```python
from build123d import *

# Parameters (mm, degrees)
F0_R          = 12.7
F1_DEPTH      = 1.27
F1_DEPTH_BACK = 1.27
F0_W          = 2.54
F0_H          = 2.54
F2_DEPTH      = 10.16
F2_DEPTH_BACK = 10.16
F3_DEPTH      = 1.27
F3_DEPTH_BACK = 1.27
F4_DEPTH      = 1.27
F4_DEPTH_BACK = 1.27
F5_DEPTH      = 1.27
F5_DEPTH_BACK = 1.27
F6_DEPTH      = 1.27
F6_DEPTH_BACK = 1.27


# Not quite as in the source:
# - a feature of the source that left no trace in its solid (it failed there, or was rolled back) is left out
# - a pattern or mirror of a feature is missing from the dataset's text; its kind, count and spacing are read off the source's solid


with BuildPart() as f1:
    # F0 (on Right) → F1 (new body, two sides)
    with BuildSketch(Plane.YZ) as f1_sk:
        Circle(F0_R)
        with BuildLine():
            ThreePointArc((-10.0803124952, 1.27), (-7.1842048969, 7.1842048969), (-1.27, 10.0803124952))
            ThreePointArc((-1.27, 10.0803124952), (0, 10.16), (1.27, 10.0803124952))
            ThreePointArc((1.27, 10.0803124952), (7.1842048969, 7.1842048969), (10.0803124952, 1.27))
            ThreePointArc((10.0803124952, 1.27), (10.1400585538, 0.6362487914), (10.16, 0))
            ThreePointArc((10.16, 0), (10.1400585538, -0.6362487914), (10.0803124952, -1.27))
            ThreePointArc((10.0803124952, -1.27), (7.1842048969, -7.1842048969), (1.27, -10.0803124952))
            ThreePointArc((1.27, -10.0803124952), (0, -10.16), (-1.27, -10.0803124952))
            ThreePointArc((-1.27, -10.0803124952), (-7.1842048969, -7.1842048969), (-10.0803124952, -1.27))
            ThreePointArc((-10.0803124952, -1.27), (-10.16, 0), (-10.0803124952, 1.27))
        make_face(mode=Mode.SUBTRACT)
    extrude(amount=F1_DEPTH)
    extrude(f1_sk.sketch, amount=-F1_DEPTH_BACK)

    # F1_copies: F1 across plane


with BuildPart() as f1_1:
    add(f1.part)
    add(f1.part.mirror(Plane(origin=(0, 0, 0), x_dir=(0.7071067812, 0, -0.7071067812), z_dir=(0.7071067812, 0, 0.7071067812))))

    # F1_copies1: F1 across plane


with BuildPart() as f1_2:
    add(f1_1.part)
    add(f1_1.part.mirror(Plane(origin=(0, 0, 0), x_dir=(-0.7071067812, 0.7071067812, 0), z_dir=(-0.7071067812, -0.7071067812, 0))))

    # F0 (on Right) → F2 (join, two sides)
    with BuildSketch(Plane.YZ) as f2_sk:
        Rectangle(F0_W, F0_H)
    extrude(amount=F2_DEPTH)
    extrude(f2_sk.sketch, amount=-F2_DEPTH_BACK)

    # F0 (on Right) → F3 (join, two sides)
    with BuildSketch(Plane.YZ) as f3_sk:
        with BuildLine():
            Line((1.27, -1.27), (-1.27, -1.27))
            Line((-1.27, -1.27), (-1.27, -10.0803124952))
            ThreePointArc((-1.27, -10.0803124952), (0, -10.16), (1.27, -10.0803124952))
            Line((1.27, -10.0803124952), (1.27, -1.27))
        make_face()
    extrude(amount=F3_DEPTH)
    extrude(f3_sk.sketch, amount=-F3_DEPTH_BACK)

    # F0 (on Right) → F4 (join, two sides)
    with BuildSketch(Plane.YZ) as f4_sk:
        with BuildLine():
            Line((10.0803124952, 1.27), (1.27, 1.27))
            Line((1.27, 1.27), (1.27, -1.27))
            Line((1.27, -1.27), (10.0803124952, -1.27))
            ThreePointArc((10.0803124952, -1.27), (10.1400585538, -0.6362487914), (10.16, 0))
            ThreePointArc((10.16, 0), (10.1400585538, 0.6362487914), (10.0803124952, 1.27))
        make_face()
    extrude(amount=F4_DEPTH)
    extrude(f4_sk.sketch, amount=-F4_DEPTH_BACK)

    # F0 (on Right) → F5 (join, two sides)
    with BuildSketch(Plane.YZ) as f5_sk:
        with BuildLine():
            Line((-1.27, -1.27), (-1.27, 1.27))
            Line((-1.27, 1.27), (-10.0803124952, 1.27))
            ThreePointArc((-10.0803124952, 1.27), (-10.16, 0), (-10.0803124952, -1.27))
            Line((-10.0803124952, -1.27), (-1.27, -1.27))
        make_face()
    extrude(amount=F5_DEPTH)
    extrude(f5_sk.sketch, amount=-F5_DEPTH_BACK)

    # F0 (on Right) → F6 (join, two sides)
    with BuildSketch(Plane.YZ) as f6_sk:
        with BuildLine():
            Line((-1.27, 10.0803124952), (-1.27, 1.27))
            Line((-1.27, 1.27), (1.27, 1.27))
            Line((1.27, 1.27), (1.27, 10.0803124952))
            ThreePointArc((1.27, 10.0803124952), (0, 10.16), (-1.27, 10.0803124952))
        make_face()
    extrude(amount=F6_DEPTH)
    extrude(f6_sk.sketch, amount=-F6_DEPTH_BACK)


solid = f1_2.part
```
Check sheet for the modelled part. Datum: model origin and axes. Units: mm. A direction names the side the tool comes from. Coordinates: 2 decimals unless noted, no trailing zeros. Order: outer loops, then holes, each group sorted by start corner. A loop starts at its lowest first (then second) coordinate and runs counter-clockwise, first axis right, second up. Notation, with made-up numbers: (-38, 89.5) -> (-21, 89.5) arc R14 cw to (-21, 106.5) -> close; hole circle Ø4 at (8, 82.25). An arc over 180 degrees is marked (long way). Write item = value, one per line. Start each with the question number.
1) Go/stop test with flat-tipped pins: P1, Ø5, axis at y = -6.5, z = 5, coming from the +X side; P2, Ø5, axis at x = 4, y = 7.5, coming from the +Z side; P3, Ø0.8, axis at y = -7.5, z = 0, coming from the -X side. Record where each tip stops, or that it passes through.
2) Cross-section at A-A (x = -2.25). Enter the section's corners in (y, z).
3) Access from +Z, -Z, +X, -X, +Y, -Y to the whole of each face (thin tool, end or side, straight path). Record for faces 4 (the cylindrical face through (0.8, 12.7, 0)), 5 (the flat face through (-7.4, -7.4, 1.27)), 6 (the flat face through (7.4, 1.27, 7.4)).
4) Mould release check, pull along Y, two halves, no side actions. Record for faces 1 (the cylindrical face through (0.8, 0, 12.7)), 2 (the cylindrical face through (7.25, -7.12, -0.02)), 3 (the cylindrical face through (9.07, -0.02, -8.89)): +Y half, -Y half, draft (parallel to the pull), parting line (faces both ways), or undercut.
5) Cross-section at C-C (z = -10.5). Enter the section's corners in (x, y).
6) Material ranges on L1, parallel to X at y = -6.25, z = -0.25; L2, parallel to Y at x = -0.5, z = -5; L3, parallel to X at y = 1, z = 9, recorded low to high.
7) Cross-section at B-B (y = 9). Enter the section's corners in (x, z), then the cut area to 3 significant figures.
Ans:
q1.P1 = 1.27
q1.P2 = 1.27
q1.P3 = -10.53
q2.outline = (-12.5, -1.27) -> (-9.91, -1.27) -> (-9.91, 1.27) -> (-12.5, 1.27) -> close; (-1.27, -12.5) -> (1.27, -12.5) -> (1.27, -9.91) -> (-1.27, -9.91) -> close; (-1.27, -1.27) -> (1.27, -1.27) -> (1.27, 1.27) -> (-1.27, 1.27) -> close; (-1.27, 9.91) -> (1.27, 9.91) -> (1.27, 12.5) -> (-1.27, 12.5) -> close; (9.91, -1.27) -> (12.5, -1.27) -> (12.5, 1.27) -> (9.91, 1.27) -> close
q3.face_4 = +X, +Y
q3.face_5 = +Z, -X, -Y
q3.face_6 = +Z, +X, +Y
q4.face_1 = parting line
q4.face_2 = undercut
q4.face_3 = draft
q5.outline = (-7.14, -1.27) -> (-1.27, -1.27) -> (-1.27, -7.14) -> (1.27, -7.14) -> (1.27, -1.27) -> (7.14, -1.27) -> (7.14, 1.27) -> (1.27, 1.27) -> (1.27, 7.14) -> (-1.27, 7.14) -> (-1.27, 1.27) -> (-7.14, 1.27) -> close
q6.L1 = -11.06 to -8.01, -1.27 to 1.27, 8.01 to 11.06
q6.L2 = -11.67 to -8.84, -1.27 to 1.27, 8.84 to 11.67
q6.L3 = -8.96 to -4.71, -1.27 to 1.27, 4.71 to 8.96
q7.outline = (-8.96, -1.27) -> (-4.71, -1.27) -> (-4.71, 1.27) -> (-8.96, 1.27) -> close; (-1.27, -8.96) -> (1.27, -8.96) -> (1.27, -4.71) -> (-1.27, -4.71) -> close; (-1.27, -1.27) -> (1.27, -1.27) -> (1.27, 1.27) -> (-1.27, 1.27) -> close; (-1.27, 4.71) -> (1.27, 4.71) -> (1.27, 8.96) -> (-1.27, 8.96) -> close; (4.71, -1.27) -> (8.96, -1.27) -> (8.96, 1.27) -> (4.71, 1.27) -> close
q7.area = 49.6 mm²
